The drawing under review shows one solid part. Ordinate dimensions are in mm from its lowest x, y, z. A direction names the side the tool comes from. Give positions to 0.01 mm unless a question says otherwise; leave off trailing zeros. Order: outer loops, then holes, each group sorted by start corner. A loop starts at its lowest first (then second) coordinate and runs counter-clockwise, first axis right, second up. Notation, with made-up numbers: (76.25, 85.25) -> (135.25, 85.25) arc R27 ccw to (135.25, 107.25) -> close; hole circle Ø10 at (87, 8.5). An arc over 180 degrees is marked (long way). Return JSON: item names as keys, results as strings. Group by question number.
1) Add section A-A (x = 70.5). Give the boundary of the cut face in (y, z), then the cut area to 3 significant figures.
2) The part is to be moulded in two halves that separate along Y. For the marked faces 3, 4 and 5, say which applies: released by +Y, released by -Y, zero draft, split by the parting line, or undercut.
3) For the marked faces 1 and 2, list the 3-axis set-ups (+Z, -Z, +X, -X, +Y, -Y) from which the entire face can be reached by the end or side of a thin tool; tool diameter is ignored.
4) Add section C-C (z = 103.5). Give the boundary of the cut face in (x, y), then the cut area to 3 significant figures.
5) Insertion check: P1, Ø5, axis at x = 108, y = 67.5, coming from the -Z side; P2, Ø12, axis at x = 115, z = 81, coming from the +Y side. Each pin has a flat end and moves straight along its axis. Give the tip position at first contact, or say it passes through.
6) Add section D-D (x = 38.5). Give the boundary of the cut face in (y, z).
7) Add section B-B (y = 69). Give the boundary of the cut face in (x, z) (1 decimal), then the cut area to 3 significant figures.
8) To check wall thickness, follow line 1 along Z through (x, y) = (49.5, 29.5); line 2 along Y through (x, z) = (96.5, 52.5); line 3 along Y through (x, z) = (80, 111). State the ranges of each line that lie inside material, in increasing order.
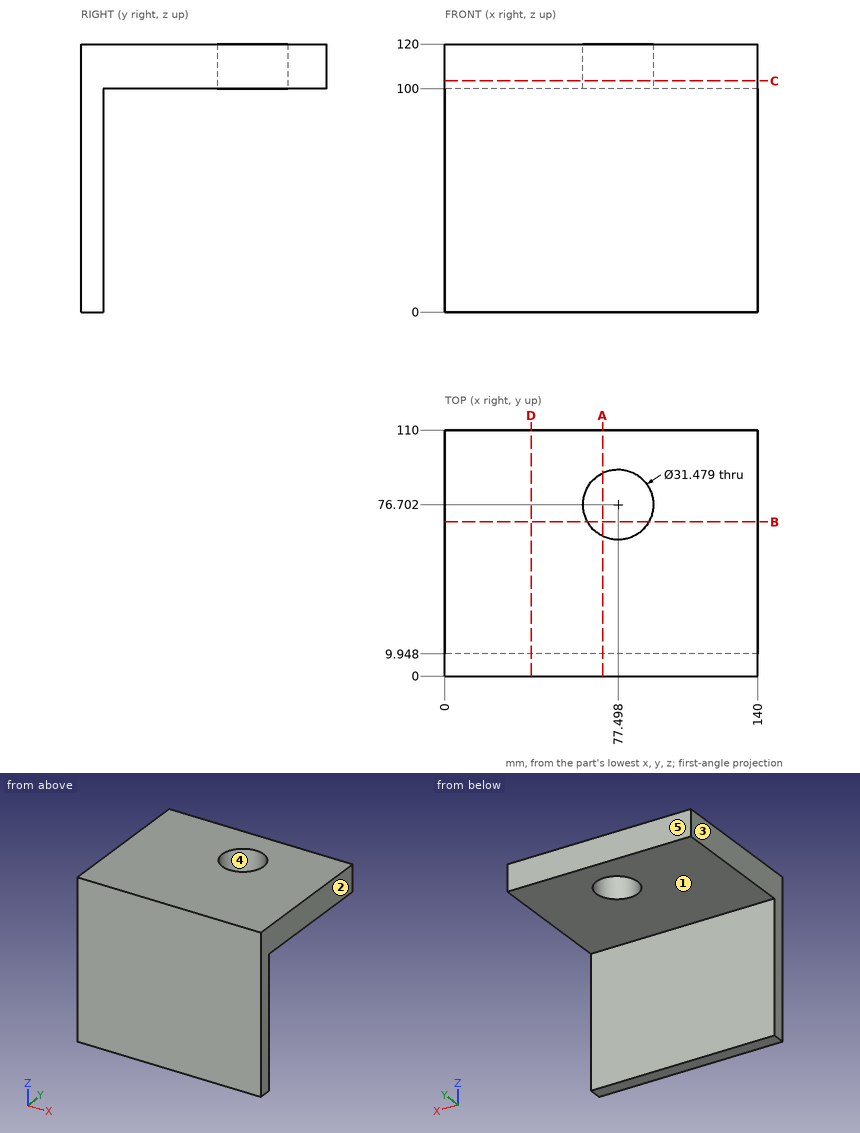
Evaluation:
{
 "1": {"outline": "(0, 0) -> (9.95, 0) -> (9.95, 100) -> (62.6, 100) -> (62.6, 120) -> (0, 120) -> close; (90.8, 100) -> (110, 100) -> (110, 120) -> (90.8, 120) -> close", "area": "2,630 mm^2"},
 "2": {"face 3": "zero draft", "face 4": "undercut", "face 5": "released by +Y"},
 "3": {"face 1": "-Z, +X, -X, +Y", "face 2": "+Z, -Z, +X, +Y, -Y"},
 "4": {"outline": "(0, 0) -> (140, 0) -> (140, 110) -> (0, 110) -> close; hole circle Ø31.48 at (77.5, 76.7)", "area": "14,600 mm^2"},
 "5": {"P1": "z = 100", "P2": "y = 9.95"},
 "6": {"outline": "(0, 0) -> (9.95, 0) -> (9.95, 100) -> (110, 100) -> (110, 120) -> (0, 120) -> close"},
 "7": {"outline": "(0, 100) -> (63.8, 100) -> (63.8, 120) -> (0, 120) -> close; (91.2, 100) -> (140, 100) -> (140, 120) -> (91.2, 120) -> close", "area": "2,250 mm^2"},
 "8": {"line 1": "100 to 120", "line 2": "0 to 9.95", "line 3": "0 to 61.16, 92.24 to 110"}
}
